Design review of the part shown in the three views and the two pictorial views. Dimensions are in mm from the part's minimum x, y and z. Coordinates: 2 decimals unless noted, no trailing zeros. Order: outer loops, then holes, each group sorted by start corner. A loop starts at its lowest first (then second) coordinate and runs counter-clockwise, first axis right, second up. Notation, with made-up numbers: (-26.5, 8) -> (11.5, 8) arc R26 cw to (11.5, 32) -> close; hole circle Ø5 at (52.5, 12). An arc over 180 degrees is marked (long way). Write item = value, one per line. Start each with the question number.
1) Wall thickness on probe 1 along X at (y, z) = (1.4, 44) (3 decimals); probe 2 along X at (y, z) = (0.65, 36): over which ranges is each line inside the solid? List them lowest first. Write a range as [from, to].
2) Consider section A-A on x = 99.5. Give the boundary of the cut face in (y, z) (3 decimals), and give its area (3 significant figures).
3) Insertion check: pin 1 Ø3 at (x, z) = (85.5, 34.5) entering from -Y. The pin has a flat end and moves straight along its axis. Give the tip position at first contact, or say it passes through.
4) Consider section B-B on z = 34.5. Give the boundary of the cut face in (x, y) (3 decimals), and give its area (3 significant figures).
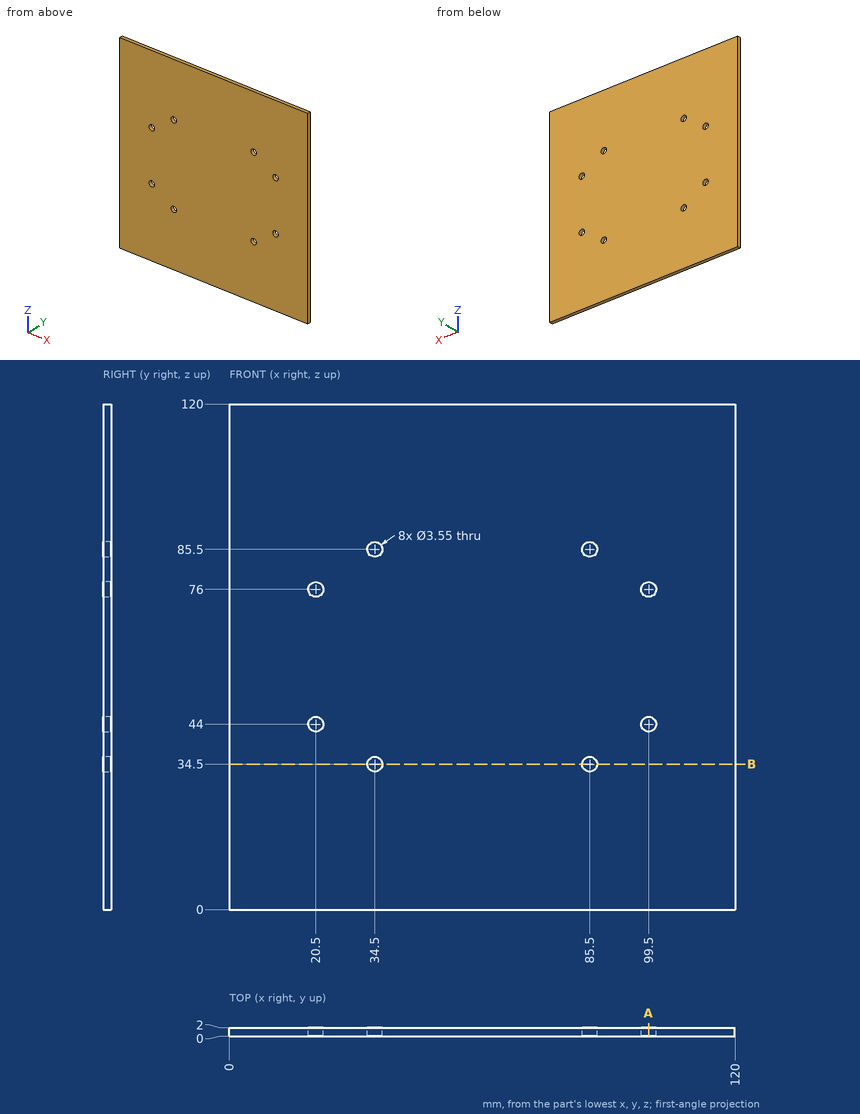
Answer sheet:
q1.probe_1 = [0, 18.725], [22.275, 97.725], [101.275, 120]
q1.probe_2 = [0, 33.55], [35.45, 84.55], [86.45, 120]
q2.outline = (0, 0) -> (2, 0) -> (2, 42.225) -> (0, 42.225) -> close; (0, 45.775) -> (2, 45.775) -> (2, 74.225) -> (0, 74.225) -> close; (0, 77.775) -> (2, 77.775) -> (2, 120) -> (0, 120) -> close
q2.area = 226 mm2
q3.pin_1 = through
q4.outline = (0, 0) -> (32.725, 0) -> (32.725, 2) -> (0, 2) -> close; (36.275, 0) -> (83.725, 0) -> (83.725, 2) -> (36.275, 2) -> close; (87.275, 0) -> (120, 0) -> (120, 2) -> (87.275, 2) -> close
q4.area = 226 mm2
